The listing builds one solid part. Answer for the finished solid, in the listing's coordinates (mm). A direction names the side the tool comes from. Round coordinates to 2 decimals unless told otherwise and drop trailing zeros. Loops run counter-clockwise (first coordinate to the right, second up) from the corner with the lowest first, then second, coordinate; pieces in that order, holes last. Notation, with made-up numbers: M 31,49.25 L 43,49.25 A26 ccw 43,82.25 Z; hole C 6.25,-4.75 d10. An arc over 180 degrees is marked long. Answer as a JSON object with one key per item and string values.
```python
from build123d import *

# Parameters (mm, degrees)
F0_W          = 1.9936040044
F0_H          = 36.5494191647
F1_DEPTH      = 2.286
F2_DEPTH      = 36.83
F3_W          = 33.3596542478
F3_H          = 0.8849272299
F4_DEPTH      = 36.5494316
F4_DEPTH_BACK = 25.4
F5_W          = 0.8558779955
F5_H          = 33.6590727701
F6_DEPTH      = 36.5494316
F7_W          = 0.9992271662
F7_H          = 33.6590727701
F8_DEPTH      = 36.5494316


with BuildPart() as f1:
    # F0 (on Top) → F1 (new body)
    with BuildSketch(Plane.XY):
        Polygon((-55.1563985646, 25.9833149612), (-56.3525594771, 25.9833149612), (-56.3525594771, -12.6926153898), (-55.1563985646, -12.6926153898), (-55.1563985646, 23.8568037748), align=None)
        with Locations((-22.793546319, 5.5820941925)):
            Rectangle(F0_W, F0_H)
        Polygon((-21.7967443168, 25.9833149612), (-55.1563985646, 25.9833149612), (-55.1563985646, 23.8568037748), (-23.7903483212, 23.8568037748), (-21.7967443168, 23.8568037748), align=None)
        with BuildLine():
            Line((-23.7903483212, 23.8568037748), (-55.1563985646, 23.8568037748))
            Line((-55.1563985646, 23.8568037748), (-55.1563985646, -12.6926153898))
            Line((-55.1563985646, -12.6926153898), (-49.7072115541, -12.6926153898))
            ThreePointArc((-49.7072115541, -12.6926153898), (-39.8056404665, 1.8860553596), (-29.904069379, -12.6926153898))
            Line((-29.904069379, -12.6926153898), (-23.7903483212, -12.6926153898))
            Line((-23.7903483212, -12.6926153898), (-23.7903483212, 23.8568037748))
        make_face()
    extrude(amount=F1_DEPTH)

    # F0 (on Top) → F2 (join)
    with BuildSketch(Plane.XY):
        Polygon((-21.7967443168, 25.9833149612), (-55.1563985646, 25.9833149612), (-55.1563985646, 23.8568037748), (-23.7903483212, 23.8568037748), (-21.7967443168, 23.8568037748), align=None)
    extrude(amount=F2_DEPTH)

    # F3 (on face) → F4 (join, two sides)
    with BuildSketch(Plane.XZ.offset(-23.8568037748)) as f4_sk:
        with Locations((-38.4765714407, 36.3875363851)):
            Rectangle(F3_W, F3_H)
    extrude(amount=F4_DEPTH)
    extrude(f4_sk.sketch, amount=-F4_DEPTH_BACK)

    # F5 (on face) → F6 (join)
    with BuildSketch(Plane.XZ.offset(-23.8568037748)):
        with Locations((-54.7284595668, 19.1155363851)):
            Rectangle(F5_W, F5_H)
    extrude(amount=F6_DEPTH)

    # F7 (on face) → F8 (join)
    with BuildSketch(Plane.XZ.offset(-23.8568037748)):
        with Locations((-22.2963578999, 19.1155363851)):
            Rectangle(F7_W, F7_H)
    extrude(amount=F8_DEPTH)


solid = f1.part
```
Item 1: Which of the six approach directions +Z, -Z, +X, -X, +Y, -Y give full straight-line access (tool end or side, diameter ignored) to faces 5 (the face through (-39, 25.983, 18)), 6 (the face through (-22.796, 6, 19)), 7 (the face through (-40.1, 1.88, 1.13))?
Values follow:
{"face 5": "-Z, +X, -X, +Y", "face 6": "-Y", "face 7": "-Z"}
Item 2: The part is cut by section D-D (y = -5). Give the vertices of the cut face in (x, z), then the cut area to 3 significant figures.
Values follow:
{"outline": "M -56.35,0 L -49.77,0 L -49.77,2.29 L -54.3,2.29 L -54.3,35.95 L -22.8,35.95 L -22.8,2.29 L -29.84,2.29 L -29.84,0 L -21.8,0 L -21.8,36.83 L -55.16,36.83 L -55.16,2.29 L -56.35,2.29 Z", "area": "125 mm^2"}
Item 3: Determine the mould class of faces 1 (the face through (-39, 23.857, 19)), 2 (the face through (-38.6, -12.693, 36.3)), 3 (the face through (-39, 6, 35.945)), 4 (the face through (-39, 37, 35.945)) for opening direction Z: released by +Z, released by -Z, zero draft, split by the parting line, or undercut.
Values follow:
{"face 1": "undercut", "face 2": "zero draft", "face 3": "undercut", "face 4": "released by -Z"}
Item 4: Straight lines are drawn through the part: line 1 (Z direction, x = -30.5, y = 21); line 2 (X direction, y = -5.5, z = 2.5); line 3 (Y direction, x = -48.5, z = 12). For each, find the intervals that lie inside material, in ascending order.
Values follow:
{"line 1": "0 to 2.29, 35.95 to 36.83", "line 2": "-55.16 to -54.3, -22.8 to -21.8", "line 3": "23.86 to 25.98"}
Item 5: The part is cut by section C-C (z = 23.5). Give the vertices of the cut face in (x, y).
Values follow:
{"outline": "M -55.16,-12.69 L -54.3,-12.69 L -54.3,23.86 L -22.8,23.86 L -22.8,-12.69 L -21.8,-12.69 L -21.8,25.98 L -55.16,25.98 Z"}
Item 6: Flat-ended cylindrical pins translate along their axes: P1, Ø4, axis at x = -30, z = 18, coming from the +Y side; P2, Ø6, axis at y = 22, z = 11, coming from the -X side; P3, Ø11.5, axis at x = -40.5, y = 33.5, coming from the -Z side. Find the tip coordinate at first contact, or state that the pin passes through.
Values follow:
{"P1": "y = 25.98", "P2": "x = -55.16", "P3": "z = 35.95"}
Item 7: The part is cut by section A-A (y = 4.5). Give the vertices of the cut face in (x, z), then the cut area to 3 significant figures.
Values follow:
{"outline": "M -56.35,0 L -21.8,0 L -21.8,36.83 L -55.16,36.83 L -55.16,2.29 L -56.35,2.29 Z; hole M -54.3,2.29 L -22.8,2.29 L -22.8,35.95 L -54.3,35.95 Z", "area": "171 mm^2"}
Item 8: The part is cut by section B-B (x = -24.5). Give the vertices of the cut face in (y, z), then the cut area to 3 significant figures.
Values follow:
{"outline": "M -12.69,0 L 25.98,0 L 25.98,35.95 L 49.26,35.95 L 49.26,36.83 L -12.69,36.83 L -12.69,35.95 L 23.86,35.95 L 23.86,2.29 L -12.69,2.29 Z", "area": "215 mm^2"}
